Can you work these out from the model? Positions are in its coordinate system, mm. A direction names the side the tool comes from. Give positions to 0.01 mm unless a question says otherwise; leave off trailing zeros. Order: outer loops, then holes, each group sorted by start corner. A loop starts at its lowest first (then second) coordinate and runs counter-clockwise, first axis right, second up.
Item 1: I want a section at A-A, the plane x = 143. Write out the boundary of the cut face in (y, z), then the cut area to 3 significant figures.
Item 2: Which directions (+Z, -Z, +X, -X, +Y, -Y) give clear straight access to the entire face, cutting with the end or side of a thin tool? Please do faces 4 (the flat face through (0, 0, 0)), 5 (the flat face through (235, 4, -3)), 6 (the cylindrical face through (120.115, 16.374, -0.751)).
Item 3: If we mould it in two halves opening along Y, with no side actions, what happens to faces 1 (the flat face through (245, -12, -12)), 2 (the cylindrical face through (240.07, 0.66, 14.985)), 3 (the cylindrical face through (120.8, 1.32, 29.97))? For each: +Y half, -Y half, draft (parallel to the pull), parting line (faces both ways), or undercut.
Item 4: If I drill on line 1 along Y through (x, z) = (239.25, 0); line 2 along Y through (x, z) = (193.5, 0); line 3 along Y through (x, z) = (190, 26), over which ranges is the centre line in solid material (lowest first)?
Item 5: I'm going to push flat-ended pins straight in: pin 1 Ø4 at (x, z) = (122.5, 0) entering from +Y; pin 2 Ø10 at (x, z) = (212.5, 14.5) entering from -Y; pin 3 Ø10 at (x, z) = (38.5, -10.5) entering from +Y. Where does each tip first touch, or does it pass through?
Item 6: I want a section at B-B, the plane x = 39. Write out the boundary of the cut face in (y, z), then the cut area to 3 significant figures.
```python
from build123d import *

# Parameters (mm, degrees)
SKETCH_1_R                = 30
EXTRUDE_1_DEPTH           = 245
CHAMFER_1_SIZE            = 1
SKETCH_2_R                = 15
CUT_EXTRUDE_1_DEPTH       = 10
HOLE_WIZARD_8_0_8_1_D     = 8
HOLE_WIZARD_8_0_8_1_DEPTH = 117.5
HOLE_WIZARD_8_0_8_1_TIP   = 2.403442476
M10X1_0_1_D               = 9
M10X1_0_1_DEPTH           = 20
M10X1_0_1_TIP             = 2.703872786
HOLE_WIZARD_5_0_5_1_D     = 5
HOLE_WIZARD_5_0_5_1_DEPTH = 30
HOLE_WIZARD_5_0_5_1_TIP   = 1.502151548


with BuildPart() as part:
    # 草图1 → 凸台-拉伸1 (new body)
    with BuildSketch(Plane(origin=(0, 0, 0), x_dir=(0, 0, -1), z_dir=(1, 0, 0))):
        Circle(SKETCH_1_R)
    extrude(amount=EXTRUDE_1_DEPTH)

    # 倒角1
    chamfer_1_edges = [part.edges().sort_by_distance(p)[0] for p in [
        (0, 0, 30),
        (245, 0, 30),
    ]]
    chamfer(chamfer_1_edges, length=CHAMFER_1_SIZE)

    # 草图2 → 切除-拉伸1 (cut)
    with BuildSketch(Plane(origin=(245, 0, 0), x_dir=(0, 0, -1), z_dir=(1, 0, 0))):
        Circle(SKETCH_2_R)
    extrude(amount=-CUT_EXTRUDE_1_DEPTH, mode=Mode.SUBTRACT)

    # Ø8.0 (8) 直径孔1
    with Locations(Plane(origin=(235, 0, 0), x_dir=(0, 0, -1), z_dir=(1, 0, 0))):
        with Locations((0, 0)):
            Hole(HOLE_WIZARD_8_0_8_1_D / 2, depth=HOLE_WIZARD_8_0_8_1_DEPTH)
            with Locations((0, 0, -(HOLE_WIZARD_8_0_8_1_DEPTH + HOLE_WIZARD_8_0_8_1_TIP / 2))):  # 118° drill point
                Cone(0, HOLE_WIZARD_8_0_8_1_D / 2, HOLE_WIZARD_8_0_8_1_TIP, mode=Mode.SUBTRACT)

    # M10x1.0 螺纹孔1
    with Locations(Plane(origin=(235, 0, 0), x_dir=(0, 0, -1), z_dir=(1, 0, 0))):
        with Locations((0, 0)):
            Hole(M10X1_0_1_D / 2, depth=M10X1_0_1_DEPTH)
            with Locations((0, 0, -(M10X1_0_1_DEPTH + M10X1_0_1_TIP / 2))):  # 118° drill point
                Cone(0, M10X1_0_1_D / 2, M10X1_0_1_TIP, mode=Mode.SUBTRACT)

    # Ø5.0 (5) 直径孔1
    with Locations(Plane(origin=(0, 30, 0), x_dir=(1, 0, 0), z_dir=(0, 1, 0))):
        with Locations((122.5, 0)):
            Hole(HOLE_WIZARD_5_0_5_1_D / 2, depth=HOLE_WIZARD_5_0_5_1_DEPTH)
            with Locations((0, 0, -(HOLE_WIZARD_5_0_5_1_DEPTH + HOLE_WIZARD_5_0_5_1_TIP / 2))):  # 118° drill point
                Cone(0, HOLE_WIZARD_5_0_5_1_D / 2, HOLE_WIZARD_5_0_5_1_TIP, mode=Mode.SUBTRACT)


solid = part.part
```
Results list:
1. outline: circle Ø60 at (0, 0); hole circle Ø8 at (0, 0)
1. area: 2,780 mm2
2. face 4: +Z, -Z, -X, +Y, -Y
2. face 5: +X
2. face 6: +Y
3. face 1: draft
3. face 2: undercut
3. face 3: parting line
4. line 1: y = -30 to -15, 15 to 30
4. line 2: y = -30 to -4, 4 to 30
4. line 3: y = -14.97 to 14.97
5. pin 1: stops at y = -3.46
5. pin 2: stops at y = -28.46
5. pin 3: stops at y = 29.49
6. outline: circle Ø60 at (0, 0)
6. area: 2,830 mm2
